Autodesk Inventor part; units mm, degrees
ref_plane "YZ Plane" through (0, 0, 0) normal (1, 0, 0) x (0, 1, 0)
ref_plane "XZ Plane" through (0, 0, 0) normal (0, 1, 0) x (-1, 0, 0)
ref_plane "XY Plane" through (0, 0, 0) normal (0, 0, 1) x (1, 0, 0)
sketch "スケッチ2" plane through (0, 0, 0) normal (0, 1, 0) x (-1, 0, 0)
  circle A0 centre (0, 0) radius 2
  line L0 (-6, 5) -> (6, 5)
  line L1 (6, 5) -> (6, -5)
  line L2 (6, -5) -> (-6, -5)
  line L3 (-6, -5) -> (-6, 5)
  line L4 (-6, 5) -> (6, -5) construction
  line L5 (6, 5) -> (-6, -5) construction
  line L6 (-18, 5) -> (-6, 5)
  line L7 (-6, 5) -> (-6, -5)
  line L8 (-6, -5) -> (-18, -5)
  line L9 (-18, -5) -> (-18, 5)
  line L10 (-18, 5) -> (-6, -5) construction
  line L11 (-6, 5) -> (-18, -5) construction
  point P0 (-12, 0)
  dimension "d0" = 4
  dimension "d1" = 12
  dimension "d2" = 10
  dimension "d3" = 12
extrude "押し出し1" add sketch "スケッチ2" along normal blind 4 contours A0 | L0 L1 L2 L3 | L3 L8 L9 L6
extrude "押し出し2" add sketch "スケッチ2" along normal blind 9 contours A0 | L0 L1 L2 L3
extrude "押し出し3" add sketch "スケッチ2" along normal blind 65 contours A0
sketch "スケッチ3" plane through (0, 9, 0) normal (0, 1, 0) x (1, 0, 0)
  circle A0 centre (0, 0) radius 2
  circle A1 centre (0, 0) radius 3
  dimension "d10" = 6
extrude "押し出し4" add sketch "スケッチ3" along normal blind 1 contours A0 | A1
sketch "スケッチ4" plane through (0, 4, 0) normal (0, 1, 0) x (1, 0, 0)
  circle A0 centre (12, 0) radius 6
  line L0 (18, -5) -> (18, 5)
  line L1 (6, -5) -> (6, 5)
  line L2 (6, 5) -> (6, -5)
  line L3 (6, -5) -> (18, -5)
  line L4 (18, -5) -> (18, 5)
  line L5 (18, 5) -> (6, 5)
  point P0 (0, 0)
  point P1 (15.3166, 5)
  point P2 (8.6834, 5)
  point P3 (8.6834, -5)
  point P4 (15.3166, -5)
extrude "押し出し5" add sketch "スケッチ4" along normal blind 15 contours A0 L3 L5
sketch "スケッチ5" plane through (0, 19, 0) normal (0, 1, 0) x (1, 0, 0)
  arc A0 (8.6834, 5) -> (8.6834, -5) centre (12, 0) ccw
  circle A1 centre (12, 0) radius 2
  line L0 (8.3, 2) -> (8.5, 2)
  line L1 (8.5, 2) -> (8.5, -2)
  line L2 (8.5, -2) -> (8.3, -2)
  line L3 (8.3, -2) -> (8.3, 2)
  line L4 (15.5, 2) -> (15.7, 2)
  line L5 (15.7, 2) -> (15.7, -2)
  line L6 (15.7, -2) -> (15.5, -2)
  line L7 (15.5, -2) -> (15.5, 2)
  line L8 (15.3166, 5) -> (8.6834, 5)
  line L9 (12, 5) -> (12, 0)
  line L10 (-6, -5) -> (18, -5)
  point P0 (0, 0)
  point P1 (8.5, 0)
  point P2 (15.5, 0)
  dimension "d15" = 4
  dimension "d16" = 0.2
  dimension "d17" = 3.5
extrude "押し出し6" add sketch "スケッチ5" along normal blind 1
sketch "スケッチ6" plane through (0, 4, 0) normal (0, 1, 0) x (1, 0, 0)
  line L0 (15.5, -2) -> (15.5, 2)
  line L1 (15.5, 2) -> (15.7, 2)
  line L2 (15.7, 2) -> (15.7, -2)
  line L3 (15.7, -2) -> (15.5, -2)
  line L4 (8.3, -2) -> (8.3, 2)
  line L5 (8.3, 2) -> (8.5, 2)
  line L6 (8.5, 2) -> (8.5, -2)
  line L7 (8.5, -2) -> (8.3, -2)
  circle A0 centre (12, 0) radius 2
  arc A1 (8.6834, 5) -> (8.6834, -5) centre (12, 0) ccw
  line L8 (8.6834, -5) -> (15.3166, -5)
  arc A2 (15.3166, -5) -> (15.3166, 5) centre (12, 0) ccw
  line L9 (15.3166, 5) -> (8.6834, 5)
  circle A3 centre (12, 0) radius 5.5
  line L10 (15.1623, -4.5) -> (8.8377, -4.5)
  line L11 (8.8377, -4.5) -> (8.8377, 4.5)
  line L12 (8.8377, 4.5) -> (15.1623, 4.5)
  line L13 (15.1623, 4.5) -> (15.1623, -4.5)
  line L14 (15.1623, -4.5) -> (8.8377, 4.5) construction
  line L15 (8.8377, -4.5) -> (15.1623, 4.5) construction
  point P0 (0, 0)
  dimension "d20" = 11
  dimension "d21" = 9
extrude "押し出し7" cut sketch "スケッチ6" along normal blind 0.2 contours L9 A3 L8 A1 | L9 A3 L12 | A3 L10 L8 | L9 A2 L8 A3
sketch "スケッチ7" plane through (0, 0, 0) normal (0, -1, 0) x (1, 0, 0)
  line L0 (17.5, -4.5) -> (-5.5, -4.5)
  line L1 (-5.5, -4.5) -> (-5.5, 4.5)
  line L2 (-5.5, 4.5) -> (17.5, 4.5)
  line L3 (17.5, 4.5) -> (17.5, -4.5)
  line L4 (6, -5) -> (6, 5)
  line L5 (17.5, -4.5) -> (-5.5, 4.5) construction
  line L6 (-5.5, -4.5) -> (17.5, 4.5) construction
  line L7 (-6, -5) -> (-6, 5)
  line L8 (18, -5) -> (-6, -5)
  circle A0 centre (8, -3) radius 1.5
  circle A1 centre (16, 3) radius 1.5
  circle A2 centre (4, -3) radius 1.5
  circle A3 centre (-4, 3) radius 1.5
  line L9 (5.5, 4.5) -> (6.5, 4.5)
  line L10 (6.5, 4.5) -> (6.5, -4.5)
  line L11 (6.5, -4.5) -> (5.5, -4.5)
  line L12 (5.5, -4.5) -> (5.5, 4.5)
  line L13 (5.5, 4.5) -> (6.5, -4.5) construction
  line L14 (6.5, 4.5) -> (5.5, -4.5) construction
  line L15 (18, -5) -> (-6, -5)
  line L16 (18, 5) -> (18, -5)
  line L17 (-6, 5) -> (18, 5)
  line L18 (-6, -5) -> (-6, 5)
  point P0 (0, 0)
  point P1 (6, 0)
  dimension "d24" = 23
  dimension "d25" = 0.5
  dimension "d26" = 0.5
  dimension "d27" = 3
  dimension "d31" = 1
extrude "押し出し8" cut sketch "スケッチ7" against normal blind 3 contours L3 L2 L4 L17 L16 L8 L0 | L0 A0 L10 L2 A1 L3 | L0 L10 A0 | A1 L2 L3 | L0 L4 L2 L10 | L4 L8 L7 L17 L2 L1 L0 | L0 L12 L2 L4 | L0 A2 L12 | L0 L1 A3 L2 L12 A2 | A3 L1 L2
extrude "押し出し9" add sketch "スケッチ2" along normal blind 0.5 contours A0 | L0 L1 L2 L3 | L3 L8 L9 L6
sketch "スケッチ9" plane through (0, 0, 0) normal (0, -1, 0) x (1, 0, 0)
  circle A0 centre (4, -3) radius 1.5
  circle A1 centre (4, -3) radius 1.5
  circle A2 centre (4, 2) radius 3
  line L0 (-6, 5) -> (18, 5)
  point P0 (0, 0)
  dimension "d38" = 6
extrude "押し出し10" add sketch "スケッチ9" against normal up to surface (3 mm away) contours A2
equation "\"d26\" = d25"
properties part number "motor_M4_55" material "アルミニウム 6061"
The model under review builds one solid part; all positions refer to its coordinate system, in mm. A direction names the side the tool comes from. Round coordinates to 2 decimals unless told otherwise and drop trailing zeros. Loops run counter-clockwise (first coordinate to the right, second up) from the corner with the lowest first, then second, coordinate; pieces in that order, holes last.
Item 1: For line 1 (Y direction, x = 14, z = 4.75); line 2 (Y direction, x = 0, z = 4.25); line 3 (Y direction, x = 17, z = -0.25), list the stretches that pass through material, from the lowest coordinate up.
Determined:
line 1: y = 0 to 0.5, 3 to 4, 4.2 to 19
line 2: y = 0 to 0.5, 3 to 9
line 3: y = 0 to 0.5, 3 to 19
Item 2: Mouldability with a two-part tool opening along X and no side actions: class faces 1 (the face through (6.89, 1.73, -1.99)), 2 (the face through (7, 4, 4)), 3 (the face through (12, 20, 0)) as released by +X, released by -X, zero draft, split by the parting line, or undercut.
Determined:
face 1: undercut
face 2: undercut
face 3: zero draft
Item 3: Take a section at A-A (y = 35). Write out the cut boundary in (x, z), then the cut area to 3 significant figures.
Determined:
outline: circle Ø4 at (0, 0)
area: 12.6 mm2
Item 4: Clearance check with flat-ended pins moving along their axes: pin 1 Ø10 at (x, y) = (3.5, 29.5) entering from -Z; pin 2 Ø1.2 at (x, z) = (13, 0) entering from +Y; pin 3 Ø3 at (y, z) = (12.5, -3) entering from -X. State where each tip first meets the part, or that it passes through.
Determined:
pin 1: stops at z = -2
pin 2: stops at y = 20
pin 3: stops at x = -1.32
Item 5: For faces 4 (the face through (14.5, 1.73, 3.07)), 5 (the face through (9, 9, -5)), 6 (the face through (17, 4, 4)), 7 (the face through (-3, 9.5, 0.1)), list the 3-axis set-ups (+Z, -Z, +X, -X, +Y, -Y) from which the entire face can be reached by the end or side of a thin tool; tool diameter is ignored.
Determined:
face 4: none
face 5: -Z, +X, -X, +Y, -Y
face 6: +Z, +X, +Y
face 7: +Y
